The model under review builds one solid part; all positions refer to its coordinate system, in mm. A direction names the side the tool comes from. Round coordinates to 2 decimals unless told otherwise and drop trailing zeros. Order: outer loops, then holes, each group sorted by start corner. A loop starts at its lowest first (then second) coordinate and runs counter-clockwise, first axis right, second up. Notation, with made-up numbers: M -38,41 L -29,41 A23 ccw -29,62 Z; hole C -6.5,87 d5. An arc over 180 degrees is marked long. Answer as a JSON object with one key per item and string values. Group by question number.
1. Add section A-A on z = 26.5. State the section outline as (x, y) points.
2. Mouldability with a two-part tool opening along Y and no side actions: class faces 1 (the face through (-29, 10, -2)), 2 (the face through (-8.01, 5.07, 28.87)), 3 (the face through (-4.37, 8.25, -13.88)) as released by +Y, released by -Y, zero draft, split by the parting line, or undercut.
3. To check wall thickness, follow probe 1 along X at (y, z) = (7.25, 0); probe 2 along Y at (x, z) = (-16, -0.5); probe 3 along X at (y, z) = (30.6, 0). State the ranges of each line that lie inside material, in increasing order. Write a range as [from, to].
4. Add section C-C on y = 27. State the section outline as (x, z) points, and give its area (3 significant figures).
5. Add section B-B on z = 0. Give the number of separate pieces and of enclosed holes in the cut face, and give its area (3 significant figures).
6. Add section D-D on y = 20. State the section outline as (x, z) points, and give its area (3 significant figures).
7. Clearance check with flat-ended pins moving along their axes: P1, Ø8, axis at x = 18, y = 20, coming from the -Z side; P2, Ø14.5, axis at x = 6, z = -1, coming from the -Y side; P3, Ø6.5, axis at x = -11.5, z = -28, coming from the +Y side. State where each tip first meets the part, or that it passes through.
8. Machinability: for faces 4 (the face through (21, 5.07, 21.37)), 5 (the face through (4.46, 4.93, 25)), 6 (the face through (-20.987, 5.07, 21.351)), 7 (the face through (-29, 5, -7.5)), which of the approach directions +Z, -Z, +X, -X, +Y, -Y give a long, thin tool a straight path to every point of the face, cutting with its end or side? Answer none if there is none.
```python
from build123d import *

# Parameters (mm, degrees)
CHAMFER1_SIZE          = 0.3
CUT_EXTRUDE4_START     = 10.66266842
CUT_EXTRUDE4_OUTLINE_R = 2.9
CUT_EXTRUDE4_DEPTH     = 13.33733168
BOSS_EXTRUDE1_START    = -10
SKETCH10_R             = 1.8
BOSS_EXTRUDE1_DEPTH    = 10
FILLET1_R              = 8
SKETCH11_R             = 14.05
BOSS_EXTRUDE2_DEPTH    = 0.1
SKETCH12_R             = 21.35
BOSS_EXTRUDE3_DEPTH    = 0.1
SKETCH13_R             = 14.35
BOSS_EXTRUDE4_DEPTH    = 0.1


# Read off the part's stored shape, not the designer's step: Cut-Extrude4
with BuildPart() as part:
    # Sketch1 → Revolve1 (revolve)
    with BuildSketch(Plane.XY, mode=Mode.PRIVATE) as revolve1_sk:
        Polygon((-14.05, 0), (-24, 0), (-24, 31.5), (-14.05, 31.5), (-14.05, 29.3), (-16.3, 29.3), (-16.3, 25.2), (-14.05, 25.2), (-14.05, 23.5), (-14.55, 23.5), (-14.55, 23), (-14.05, 23), (-11.05, 23), (-11.05, 8.5), (-14.05, 8.5), (-14.55, 8.5), (-14.55, 8), (-14.05, 8), (-14.05, 6.3), (-16.6, 6.3), (-16.6, 2.2), (-14.05, 2.2), align=None)
    revolve(revolve1_sk.sketch.rotate(Axis((0, 0, 0), (0, 1, 0)), 270), axis=Axis((0, 0, 0), (0, 1, 0)))

    # Chamfer1
    chamfer1_edges = [part.edges().sort_by_distance(p)[0] for p in [
        (0, 2.2, 16.6),
        (0, 2.2, 14.05),
        (0, 0, 14.05),
        (0, 31.5, 24),
        (0, 31.5, 14.05),
        (0, 29.3, 14.05),
        (0, 29.3, 16.3),
        (0, 25.2, 16.3),
        (0, 25.2, 14.05),
        (0, 23, 11.05),
        (0, 8.5, 11.05),
        (0, 6.3, 16.6),
    ]]
    chamfer(chamfer1_edges, length=CHAMFER1_SIZE)

    # Cut-Extrude4 outline → Cut-Extrude4 (cut)
    with BuildSketch(Plane.XY.offset(CUT_EXTRUDE4_START)):
        with Locations((0, 15.6)):
            Circle(CUT_EXTRUDE4_OUTLINE_R)
    extrude(amount=CUT_EXTRUDE4_DEPTH, mode=Mode.SUBTRACT)

    # Sketch10 → Boss-Extrude1 (add)
    # profile 1 of 6: a face of its own
    with BuildSketch(Plane.XZ.offset(BOSS_EXTRUDE1_START)):
        with BuildLine():
            Line((-30, 7.5), (-22.79802623, 7.5))
            ThreePointArc((-22.79802623, 7.5), (-24, 0), (-22.79802623, -7.5))
            Line((-22.79802623, -7.5), (-30, -7.5))
            ThreePointArc((-30, -7.5), (-37.5, 0), (-30, 7.5))
        make_face()
        with Locations(Location((-30, 0, 0), (0, 0, 270))):
            Circle(SKETCH10_R, mode=Mode.SUBTRACT)
    # profile 2 of 6: a face of its own
    with BuildSketch(Plane.XZ.offset(BOSS_EXTRUDE1_START)):
        with BuildLine():
            Line((-8.504809472, 29.730762114), (-4.903822587, 23.493669872))
            ThreePointArc((-4.903822587, 23.493669872), (-12, 20.784609691), (-17.894203644, 15.993669872))
            Line((-17.894203644, 15.993669872), (-21.495190528, 22.230762114))
            ThreePointArc((-21.495190528, 22.230762114), (-18.75, 32.475952642), (-8.504809472, 29.730762114))
        make_face()
        with Locations(Location((-15, 25.980762114, 0), (0, 0, 270))):
            Circle(SKETCH10_R, mode=Mode.SUBTRACT)
    # profile 3 of 6: a face of its own
    with BuildSketch(Plane.XZ.offset(BOSS_EXTRUDE1_START)):
        with BuildLine():
            Line((21.495190528, 22.230762114), (17.894203644, 15.993669872))
            ThreePointArc((17.894203644, 15.993669872), (12, 20.784609691), (4.903822587, 23.493669872))
            Line((4.903822587, 23.493669872), (8.504809472, 29.730762114))
            ThreePointArc((8.504809472, 29.730762114), (18.75, 32.475952642), (21.495190528, 22.230762114))
        make_face()
        with Locations(Location((15, 25.980762114, 0), (0, 0, 270))):
            Circle(SKETCH10_R, mode=Mode.SUBTRACT)
    # profile 4 of 6: a face of its own
    with BuildSketch(Plane.XZ.offset(BOSS_EXTRUDE1_START)):
        with BuildLine():
            Line((30, -7.5), (22.79802623, -7.5))
            ThreePointArc((22.79802623, -7.5), (24, 0), (22.79802623, 7.5))
            Line((22.79802623, 7.5), (30, 7.5))
            ThreePointArc((30, 7.5), (37.5, 0), (30, -7.5))
        make_face()
        with Locations(Location((30, 0, 0), (0, 0, 270))):
            Circle(SKETCH10_R, mode=Mode.SUBTRACT)
    # profile 5 of 6: a face of its own
    with BuildSketch(Plane.XZ.offset(BOSS_EXTRUDE1_START)):
        with BuildLine():
            Line((8.504809472, -29.730762114), (4.903822587, -23.493669872))
            ThreePointArc((4.903822587, -23.493669872), (12, -20.784609691), (17.894203644, -15.993669872))
            Line((17.894203644, -15.993669872), (21.495190528, -22.230762114))
            ThreePointArc((21.495190528, -22.230762114), (18.75, -32.475952642), (8.504809472, -29.730762114))
        make_face()
        with Locations(Location((15, -25.980762114, 0), (0, 0, 270))):
            Circle(SKETCH10_R, mode=Mode.SUBTRACT)
    # profile 6 of 6: a face of its own
    with BuildSketch(Plane.XZ.offset(BOSS_EXTRUDE1_START)):
        with BuildLine():
            Line((-21.495190528, -22.230762114), (-17.894203644, -15.993669872))
            ThreePointArc((-17.894203644, -15.993669872), (-12, -20.784609691), (-4.903822587, -23.493669872))
            Line((-4.903822587, -23.493669872), (-8.504809472, -29.730762114))
            ThreePointArc((-8.504809472, -29.730762114), (-18.75, -32.475952642), (-21.495190528, -22.230762114))
        make_face()
        with Locations(Location((-15, -25.980762114, 0), (0, 0, 270))):
            Circle(SKETCH10_R, mode=Mode.SUBTRACT)
    extrude(amount=BOSS_EXTRUDE1_DEPTH)

    # Fillet1
    fillet1_edges = [part.edges().sort_by_distance(p)[0] for p in [
        (-4.903822587, 5, 23.493669872),
        (-17.894203644, 5, 15.993669872),
        (17.894203644, 5, 15.993669872),
        (4.903822587, 5, 23.493669872),
        (22.79802623, 5, -7.5),
        (22.79802623, 5, 7.5),
        (4.903822587, 5, -23.493669872),
        (17.894203644, 5, -15.993669872),
        (-17.894203644, 5, -15.993669872),
        (-4.903822587, 5, -23.493669872),
        (-22.79802623, 5, 7.5),
        (-22.79802623, 5, -7.5),
    ]]
    fillet(fillet1_edges, radius=FILLET1_R)

    # Sketch11 → Boss-Extrude2 (add)
    with BuildSketch(Plane.XZ.offset(-6.3)):
        with Locations(Location((0, 0, 0), (0, 0, 270))):
            Circle(SKETCH11_R)
    extrude(amount=-BOSS_EXTRUDE2_DEPTH)

    # Sketch12 → Boss-Extrude3 (add)
    with BuildSketch(Plane.XZ.offset(-8.5)):
        Circle(SKETCH12_R)
    extrude(amount=-BOSS_EXTRUDE3_DEPTH)

    # Sketch13 → Boss-Extrude4 (add)
    with BuildSketch(Plane.XZ.offset(-29.3)):
        Circle(SKETCH13_R)
    extrude(amount=-BOSS_EXTRUDE4_DEPTH)


solid = part.part
```
Recorded:
{
 "1": {"outline": "M -22.48,0 L -16.72,0 L -16.72,10 L -22.48,10 Z; M -13.28,0 L -6.39,0 L -6.39,10 L -13.28,10 Z; M 6.39,0 L 13.28,0 L 13.28,10 L 6.39,10 Z; M 16.72,0 L 22.48,0 L 22.48,10 L 16.72,10 Z"},
 "2": {"face 1": "released by +Y", "face 2": "zero draft", "face 3": "undercut"},
 "3": {"probe 1": "x = [-37.5, -31.8], [-28.2, -14.05], [14.05, 28.2], [31.8, 37.5]", "probe 2": "y = [0, 2.2], [6.3, 25.21], [29.29, 31.5]", "probe 3": "x = [-24, -14.05], [14.05, 24]"},
 "4": {"outline": "C 0,0 d48; hole C 0,0 d32.6", "area": "975 mm²"},
 "5": {"separate pieces": "3", "enclosed holes": "2", "area": "879 mm²"},
 "6": {"outline": "C 0,0 d48; hole C 0,0 d22.1", "area": "1,430 mm²"},
 "7": {"P1": "stops at z = -19.49", "P2": "stops at y = 6.3", "P3": "stops at y = 10"},
 "8": {"face 4": "+X, +Y, -Y", "face 5": "+Z, +Y, -Y", "face 6": "-X, +Y, -Y", "face 7": "-Z, -X, +Y, -Y"}
}
